```python
from build123d import *

# Parameters (mm, degrees)
SKETCH_1_R      = 1.45
EXTRUDE_1_DEPTH = 3
FILLET_1_R      = 3


with BuildPart() as part:
    # 草图1 → 凸台-拉伸1 (new body)
    with BuildSketch(Plane(origin=(0, 0, 0), x_dir=(1, 0, 0), z_dir=(0, 1, 0))):
        Polygon((-35, -7.5), (35, -7.5), (35, 37.5), (20, 37.5), (4.673782914, 27.382671433), (-20, 52.5), (-35, 52.5), align=None)
        with Locations(Location((-27.5, 37.5, 0), (0, 0, 270))):
            Circle(SKETCH_1_R, mode=Mode.SUBTRACT)
        with Locations(Location((-27.5, 47.5, 0), (0, 0, 270))):
            Circle(SKETCH_1_R, mode=Mode.SUBTRACT)
        with Locations(Location((27.5, 27.5, 0), (0, 0, 270))):
            Circle(SKETCH_1_R, mode=Mode.SUBTRACT)
        with Locations(Location((27.5, 17.5, 0), (0, 0, 270))):
            Circle(SKETCH_1_R, mode=Mode.SUBTRACT)
        with Locations(Location((0, 0, 0), (0, 0, 270))):
            Circle(SKETCH_1_R, mode=Mode.SUBTRACT)
        with Locations(Location((10, 0, 0), (0, 0, 270))):
            Circle(SKETCH_1_R, mode=Mode.SUBTRACT)
        with Locations(Location((-10, 0, 0), (0, 0, 270))):
            Circle(SKETCH_1_R, mode=Mode.SUBTRACT)
        Polygon((-20, 7.5), (20, 7.5), (4.264852248, 23.518008974), align=None, mode=Mode.SUBTRACT)
        Polygon((-20, 48.219055775), (2.122729676, 25.698639186), (-20, 11.094714181), align=None, mode=Mode.SUBTRACT)
        Polygon((20, 33.905285819), (6.815905486, 25.202041221), (20, 11.780944225), align=None, mode=Mode.SUBTRACT)
    extrude(amount=EXTRUDE_1_DEPTH)

    # 圆角1
    fillet_1_edges = [part.edges().sort_by_distance(p)[0] for p in [
        (-20, 1.5, -7.5),
        (20, 1.5, -7.5),
        (4.264852248, 1.5, -23.518008974),
        (2.122729676, 1.5, -25.698639186),
        (-20, 1.5, -48.219055775),
        (-20, 1.5, -11.094714181),
        (20, 1.5, -37.5),
        (35, 1.5, -37.5),
        (35, 1.5, 7.5),
        (-35, 1.5, 7.5),
        (-35, 1.5, -52.5),
        (-20, 1.5, -52.5),
        (4.673782914, 1.5, -27.382671433),
        (20, 1.5, -33.905285819),
        (6.815905486, 1.5, -25.202041221),
        (20, 1.5, -11.780944225),
    ]]
    fillet(fillet_1_edges, radius=FILLET_1_R)


solid = part.part
```
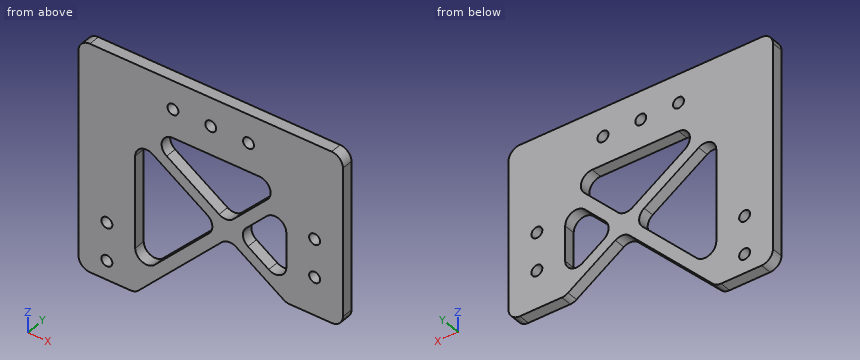
Geometry: final body of the model. Coordinates: model frame, mm. Round coordinates to 2 decimals unless told otherwise and drop trailing zeros. Order: outer loops, then holes, each group sorted by start corner. A loop starts at its lowest first (then second) coordinate and runs counter-clockwise, first axis right, second up. Notation, with made-up numbers: (-24, 31.25) -> (35, 31.25) arc R20 cw to (35, 36.25) -> close; hole circle Ø9 at (-39.75, 70.25). An arc over 180 degrees is marked (long way). Use CSV: the item, a comma, the result in double quotes. Start each with the question number.
1) First-contact query: pin 1 Ø1 at (x, y) = (11, 2) entering from -Z; pin 2 Ø4 at (x, z) = (-27.5, -47.5) entering from -Y; pin 3 Ø0.9 at (x, y) = (27, 1.5) entering from -Z. Flat tips, straight axial feed; report the tip coordinate or a pass-through.
2) Section A-A (x = 27.5). Return the cut outline in (y, z).
3) Material intervals for line 1 along X through (y, z) = (0.9, 0); line 2 along Z through (x, y) = (-12, 2.4); line 3 along Z through (x, y) = (26.5, 1.9), sorted ascending. Write a range as from..to.
4) Section B-B (z = -11). Return the cut outline in (x, y), and give its area (3 significant figures).
5) Section D-D (z = -47). Return the cut outline in (x, y).
6) Section C-C (y = 1.25). State how many separate pieces and enclosed holes the cut face has, and give its area (3 significant figures).
Returned:
1,pin 1,"stops at z = -31.89"
1,pin 2,"stops at y = 0"
1,pin 3,"stops at z = -37.5"
2,outline,"(0, -37.5) -> (3, -37.5) -> (3, -28.95) -> (0, -28.95) -> close; (0, -26.05) -> (3, -26.05) -> (3, -18.95) -> (0, -18.95) -> close; (0, -16.05) -> (3, -16.05) -> (3, 7.5) -> (0, 7.5) -> close"
3,line 1,"x = -35..-11.45, -8.55..-1.45, 1.45..8.55, 11.45..35"
3,line 2,"z = -44.36..-40.08, -16.38..-12.74, -8.26..7.5"
3,line 3,"z = -37.5..-28.55, -26.45..-18.55, -16.45..7.5"
4,outline,"(-35, 0) -> (-12.97, 0) -> (-12.97, 3) -> (-35, 3) -> close; (15.81, 0) -> (35, 0) -> (35, 3) -> (15.81, 3) -> close"
4,area,"124 mm²"
5,outline,"(-35, 0) -> (-28.86, 0) -> (-28.86, 3) -> (-35, 3) -> close; (-26.14, 0) -> (-14.6, 0) -> (-14.6, 3) -> (-26.14, 3) -> close"
6,separate pieces,"1"
6,enclosed holes,"10"
6,area,"2,500 mm²"
